```python
from build123d import *

# Parameters (mm, degrees)
SKETCH_2_W          = 114
SKETCH_2_H          = 45
EXTRUDE_1_DEPTH     = 3
SKETCH_3_W          = 5
SKETCH_3_H          = 15
CUT_EXTRUDE_1_DEPTH = 10


with BuildPart() as part:
    # 草图2 → 凸台-拉伸1 (new body)
    with BuildSketch(Plane.XY):
        Polygon((60, 67), (60, 0), (-60, 0), (-60, 67), (-100, 67), (-100, -93), (-57, -93), (-57, -83), (57, -83), (57, -93), (100, -93), (100, 67), align=None)
        with Locations((0, -45.5)):
            Rectangle(SKETCH_2_W, SKETCH_2_H, mode=Mode.SUBTRACT)
    extrude(amount=EXTRUDE_1_DEPTH)

    # 草图3 → 切除-拉伸1 (cut)
    with BuildSketch(Plane.XY.offset(3)):
        with Locations((-77.5, -48.5)):
            Rectangle(SKETCH_3_W, SKETCH_3_H)
        with Locations((77.5, -48.5)):
            Rectangle(SKETCH_3_W, SKETCH_3_H)
    extrude(amount=-CUT_EXTRUDE_1_DEPTH, mode=Mode.SUBTRACT)


solid = part.part
```
Input: part model. Units: mm. Frame: model coordinates. Give positions to 0.01 mm unless a question says otherwise; leave off trailing zeros. Loops run counter-clockwise (first coordinate to the right, second up) from the corner with the lowest first, then second, coordinate; pieces in that order, holes last.
1) Line query: L1, parallel to X at y = -66, z = 0.25; L2, parallel to X at y = 10, z = 1.5; L3, parallel to Y at x = 11, z = 0.7. Output: solid intervals per line, ascending.
A:
L1: x = -100 to -57, 57 to 100
L2: x = -100 to -60, 60 to 100
L3: y = -83 to -68, -23 to 0
2) Section query A-A on y = -62. Return the cut outline in (x, z).
A:
outline: (-100, 0) - (-57, 0) - (-57, 3) - (-100, 3) - close; (57, 0) - (100, 0) - (100, 3) - (57, 3) - close
3) Contact query for flat-ended pins moving along their axis: pin 1 (0.9 mm diameter, centred on x = 4.5, z = 1.5, fed in from -Y); pin 2 (0.9 mm diameter, centred on x = 9, z = 1.5, fed in from +Y). Output: stop coordinate, or through.
A:
pin 1: stops at y = -83
pin 2: stops at y = 0
4) Section query C-C on x = 14. Return the cut outline in (y, z), and give its area (3 significant figures).
A:
outline: (-83, 0) - (-68, 0) - (-68, 3) - (-83, 3) - close; (-23, 0) - (0, 0) - (0, 3) - (-23, 3) - close
area: 114 mm2
5) Section query B-B on z = 1.55. Return the cut outline in (x, y).
A:
outline: (-100, -93) - (-57, -93) - (-57, -83) - (57, -83) - (57, -93) - (100, -93) - (100, 67) - (60, 67) - (60, 0) - (-60, 0) - (-60, 67) - (-100, 67) - close; hole (-80, -56) - (-75, -56) - (-75, -41) - (-80, -41) - close; hole (-57, -68) - (57, -68) - (57, -23) - (-57, -23) - close; hole (75, -56) - (80, -56) - (80, -41) - (75, -41) - close
